from build123d import *

# Parameters (mm, degrees)
SKETCH1_W               = 22
SKETCH1_H               = 28
BOSS_EXTRUDE1_DEPTH     = 3
SKETCH2_R               = 1.45
CUT_EXTRUDE1_DEPTH      = 4
SKETCH3_W               = 28
SKETCH3_H               = 80
SKETCH3_H_2             = 3
BOSS_EXTRUDE2_DEPTH     = 2
SKETCH4_R               = 2.25
SKETCH4_W               = 22
SKETCH4_H               = 42
CUT_EXTRUDE2_DEPTH      = 10
SKETCH5_R               = 11.025
CUT_EXTRUDE3_DEPTH      = 10
SKETCH6_R               = 11.025
SKETCH6_R_2             = 9.025
BOSS_EXTRUDE3_DEPTH     = 0.5
SKETCH7_R               = 13.025
SKETCH7_R_2             = 11.025
BOSS_EXTRUDE4_DEPTH     = 5.5
SKETCH9_W               = 1.25
SKETCH9_H               = 4
CUT_EXTRUDE5_DEPTH      = 1
SKETCH4_4_R             = 3
CUT_EXTRUDE6_DEPTH      = 30.5
CUT_EXTRUDE6_DEPTH_BACK = 3
CHAMFER1_SIZE           = 4


with BuildPart() as part:
    # Sketch1 → Boss-Extrude1 (new body)
    with BuildSketch(Plane(origin=(0, 0, 0), x_dir=(1, 0, 0), z_dir=(0, 1, 0))):
        Rectangle(SKETCH1_W, SKETCH1_H)
    extrude(amount=BOSS_EXTRUDE1_DEPTH)

    # Sketch2 → Cut-Extrude1 (cut, through all)
    with BuildSketch(Plane.XZ):
        with Locations(Location((-7.5, 0, 0), (0, 0, 270))):  # turned: the seam where the file's is
            Circle(SKETCH2_R)
        with Locations(Location((7.5, 0, 0), (0, 0, 270))):  # turned: the seam where the file's is
            Circle(SKETCH2_R)
    extrude(amount=-CUT_EXTRUDE1_DEPTH, mode=Mode.SUBTRACT)

    # Sketch3 → Boss-Extrude2 (add)
    with BuildSketch(Plane(origin=(11, 0, 0), x_dir=(0, 0, -1), z_dir=(1, 0, 0))):
        with Locations((0, 43)):
            Rectangle(SKETCH3_W, SKETCH3_H)
        with Locations((0, 1.5)):
            Rectangle(SKETCH3_W, SKETCH3_H_2)
    boss_extrude2 = extrude(amount=BOSS_EXTRUDE2_DEPTH)

    # Sketch4 → Cut-Extrude2 (cut)
    with BuildSketch(Plane.ZY.offset(-11)):
        with Locations((-4.5, 8)):
            Circle(SKETCH4_R)
        with Locations((4.5, 8)):
            Circle(SKETCH4_R)
        with Locations((4.5, 58)):
            Circle(SKETCH4_R)
        with Locations((-4.5, 58)):
            Circle(SKETCH4_R)
        with Locations((0, 33)):
            Rectangle(SKETCH4_W, SKETCH4_H)
    extrude(amount=-CUT_EXTRUDE2_DEPTH, mode=Mode.SUBTRACT)

    # Mirror1: Boss-Extrude2 across plane
    add(boss_extrude2.mirror(Plane(origin=(0, 0, 0), x_dir=(0, 0, 1), z_dir=(1, 0, 0))))

    # Sketch5 → Cut-Extrude3 (cut)
    with BuildSketch(Plane(origin=(-11, 0, 0), x_dir=(0, 0, -1), z_dir=(1, 0, 0))):
        with Locations((0, 43)):
            Circle(SKETCH5_R)
    extrude(amount=-CUT_EXTRUDE3_DEPTH, mode=Mode.SUBTRACT)

    # Sketch6 → Boss-Extrude3 (add)
    with BuildSketch(Plane(origin=(-11, 0, 0), x_dir=(0, 0, -1), z_dir=(1, 0, 0))):
        with Locations((0, 43)):
            Circle(SKETCH6_R)
        with Locations((0, 43)):
            Circle(SKETCH6_R_2, mode=Mode.SUBTRACT)
    extrude(amount=-BOSS_EXTRUDE3_DEPTH)

    # Sketch7 → Boss-Extrude4 (add)
    with BuildSketch(Plane.ZY.offset(13)):
        with Locations((0, 43)):
            Circle(SKETCH7_R)
        with Locations(Location((0, 43, 0), (0, 0, 180))):  # turned: the seam where the file's is
            Circle(SKETCH7_R_2, mode=Mode.SUBTRACT)
    extrude(amount=BOSS_EXTRUDE4_DEPTH)

    # Sketch9 → Cut-Extrude5 (cut)
    with BuildSketch(Plane(origin=(13, 0, 0), x_dir=(0, 0, -1), z_dir=(1, 0, 0))):
        with Locations((0, 56)):
            Rectangle(SKETCH9_W, SKETCH9_H)
        with Locations((0, 10)):
            Rectangle(SKETCH9_W, SKETCH9_H)
    extrude(amount=-CUT_EXTRUDE5_DEPTH, mode=Mode.SUBTRACT)

    # Sketch4_4 → Cut-Extrude6 (cut, two sides)
    with BuildSketch(Plane.ZY.offset(-11)) as cut_extrude6_sk:
        with Locations((0, 78)):
            Circle(SKETCH4_4_R)
    extrude(amount=CUT_EXTRUDE6_DEPTH, mode=Mode.SUBTRACT)
    extrude(cut_extrude6_sk.sketch, amount=-CUT_EXTRUDE6_DEPTH_BACK, mode=Mode.SUBTRACT)

    # Chamfer1
    chamfer1_edges = [part.edges().sort_by_distance(p)[0] for p in [
        (12, 83, 14),
        (12, 83, -14),
        (-12, 83, 14),
        (-12, 83, -14),
    ]]
    chamfer(chamfer1_edges, length=CHAMFER1_SIZE)


solid = part.part
Part model, mm, in its own coordinate system. A direction names the side the tool comes from. Round coordinates to 2 decimals unless told otherwise and drop trailing zeros. Order: outer loops, then holes, each group sorted by start corner. A loop starts at its lowest first (then second) coordinate and runs counter-clockwise, first axis right, second up. Notation, with made-up numbers: (50, -12) -> (57, -12) arc R31 ccw to (57, 16) -> close; hole circle Ø2 at (8.5, 60). An arc over 180 degrees is marked (long way). Put each result on its own line as item: value.
Q1. Band-saw the part on D-D (y = 68). Give the cut face in (x, z), and give its area (3 significant figures).
From the geometry:
outline: (-13, -14) -> (-11, -14) -> (-11, 14) -> (-13, 14) -> close; (11, -14) -> (13, -14) -> (13, 14) -> (11, 14) -> close
area: 112 mm2
Q2. Pull direction Y, two halves, no side cores. Call faces 1 (the face through (11.986, 9.897, -3.29)), 2 (the face through (11, 61, 0)), 3 (the face through (12, 83, 0)): pulls with the +Y half, pulls with the -Y half, needs draft (parallel to the pull), parting line crosses it, or undercut.
From the geometry:
face 1: undercut
face 2: needs draft
face 3: pulls with the +Y half
Q3. Tool access for faces 4 (the face through (0, 3, 0)), 5 (the face through (-11.5, 33.8, 14)), 6 (the face through (11.8, 12, -0.2)), 7 (the face through (-15.712, 55.914, -1.696)): list every direction of +Z, -Z, +X, -X, +Y, -Y with a clear straight run to the whole face (end or side of a thin tool).
From the geometry:
face 4: +Z, -Z, +Y
face 5: +Z, +X, -X, +Y, -Y
face 6: +X
face 7: -X
Q4. Wall check: line 1 (Y direction, x = 12.15, z = -4.5); line 2 (Y direction, x = -12.6, z = 0) (3 decimals); line 3 (X direction, y = 55.5, z = 2). Give the ranges that are in metal, low to high. Write a range as [from, to].
From the geometry:
line 1: y = [0, 5.75], [10.25, 12], [54, 55.75], [60.25, 83]
line 2: y = [0, 31.975], [54.025, 75], [81, 83]
line 3: x = [-18.5, -11], [11, 13]
Q5. Band-saw the part on C-C (z = 4.5). State how many separate pieces and enclosed holes the cut face has, and give its area (3 significant figures).
From the geometry:
separate pieces: 5
enclosed holes: 0
area: 282 mm2
Q6. Band-saw the part on B-B (y = 25). Give the cut face in (x, z), and give its area (3 significant figures).
From the geometry:
outline: (-13, -14) -> (-11, -14) -> (-11, 14) -> (-13, 14) -> close; (11, -14) -> (13, -14) -> (13, -11) -> (11, -11) -> close; (11, 11) -> (13, 11) -> (13, 14) -> (11, 14) -> close
area: 68.0 mm2
Q7. Band-saw the part on A-A (y = 43). Give the cut face in (x, z) (3 decimals), and give its area (3 significant figures).
From the geometry:
outline: (-18.5, -13.025) -> (-13, -13.025) -> (-13, -14) -> (-11, -14) -> (-11, -9.025) -> (-11.5, -9.025) -> (-11.5, -11.025) -> (-18.5, -11.025) -> close; (-18.5, 11.025) -> (-11.5, 11.025) -> (-11.5, 9.025) -> (-11, 9.025) -> (-11, 14) -> (-13, 14) -> (-13, 13.025) -> (-18.5, 13.025) -> close; (11, -14) -> (13, -14) -> (13, -11) -> (11, -11) -> close; (11, 11) -> (13, 11) -> (13, 14) -> (11, 14) -> close
area: 47.9 mm2
Q8. Pin check, flat tips, straight feed: pin 1 Ø8 at (x, y) = (9.5, 70.5) entering from +Z; pin 2 Ø1 at (y, z) = (59, -6) entering from -X; pin 3 Ø1.5 at (y, z) = (14, 8) entering from +X; pin 4 Ø1.7 at (x, z) = (-7.5, 0) entering from +Y. Stop position of each tip, or through.
From the geometry:
pin 1: stops at z = 14
pin 2: stops at x = -13
pin 3: stops at x = -11
pin 4: passes through
